Autodesk Inventor part; units mm, degrees
ref_plane "YZ Plane" through (0, 0, 0) normal (1, 0, 0) x (0, 1, 0)
ref_plane "XZ Plane" through (0, 0, 0) normal (0, 1, 0) x (-1, 0, 0)
ref_plane "XY Plane" through (0, 0, 0) normal (0, 0, 1) x (1, 0, 0)
sketch "Sketch2" plane through (0, 0, 0) normal (0, 1, 0) x (-1, 0, 0)
  line L0 (0, 0) -> (-800, 0)
  line L1 (-800, 0) -> (-800, -600)
  line L2 (-800, -600) -> (0, -600)
  line L3 (0, -600) -> (0, 0)
  dimension "d4" = 800
  dimension "d5" = 600
extrude "Extrusion2" add sketch "Sketch2" along normal blind 18
sketch "Sketch3" plane through (0, 0, 0) normal (0, -1, 0) x (1, 0, 0)
  line L0 (0, -600) -> (0, 0)
  line L1 (800, 0) -> (800, -600)
  line L2 (0, 0) -> (800, 0)
  line L3 (800, 0) -> (800, -50)
  line L4 (800, -50) -> (0, -50)
  line L5 (0, -50) -> (0, 0)
  dimension "d8" = 50
extrude "Extrusion3" add sketch "Sketch3" along normal blind 18
sketch "Sketch4" plane through (0, 0, 0) normal (0, -1, 0) x (1, 0, 0)
  line L0 (0, -600) -> (0, 0)
  line L1 (800, 0) -> (800, -600)
  line L2 (0, -600) -> (800, -600)
  line L3 (800, -600) -> (800, -560)
  line L4 (800, -560) -> (0, -560)
  line L5 (0, -560) -> (0, -600)
  dimension "d11" = 40
extrude "Extrusion4" add sketch "Sketch4" along normal blind 18
equation "\"d5\" = Profundidad"
properties part number "tablero_chico" material "Wood (Birch)"
Here's how the part is built. I have some questions about the finished solid (model axes, mm). A direction names the side the tool comes from. Coordinates: 2 decimals unless noted, no trailing zeros. Loops run counter-clockwise (first coordinate to the right, second up) from the corner with the lowest first, then second, coordinate; pieces in that order, holes last. Notation, with made-up numbers: (8.5, 8) -> (42.5, 8) arc R34 cw to (42.5, 38) -> close; hole circle Ø6 at (55, -31.5). An arc over 180 degrees is marked (long way). Use one line per item in the form item = value. Start each with the question number.
(1) If we section it at B-B (x = 71): Please give me the cut outline in (y, z).
(2) We'd pull the mould along Z, two halves only. Please class faces 1 (the face through (406, -9, -560)), 2 (the face through (394, -18, -25)), 3 (the face through (394, 0, -600)), 4 (the face through (406, 0, -301)): pulls with the +Z half, pulls with the -Z half, needs draft (parallel to the pull), parting line crosses it, or undercut.
(3) Please list where these lines run through material, in increasing order: line 1 along Z through (x, y) = (398, -14.5); line 2 along Y through (x, z) = (88.5, -315).
(4) Will these pins go through, and if not, where does the flat tip stop? pin 1 (10 mm diameter, centred on x = 355, y = -0.5, fed in from +Z); pin 2 (8 mm diameter, centred on x = 222, z = -198, fed in from -Y).
(5) If we section it at A-A (y = -5.5): Please give me the cut outline in (x, z), then the cut area to 3 significant figures.
(6) If we section it at C-C (z = -484): Please give me the cut outline in (x, y).
(7) On a 3-axis mill with a long thin cutter (end or side, diameter ignored), from which of +Z, -Z, +X, -X, +Y, -Y can I reach the whole of each face in a straight line? I mean faces 5 (the face through (406, -9, -50)), 6 (the face through (394, -18, -580)). Say none if no direction works.
Verdict:
q1.outline = (-18, -600) -> (18, -600) -> (18, 0) -> (-18, 0) -> (-18, -50) -> (0, -50) -> (0, -560) -> (-18, -560) -> close
q2.face_1 = undercut
q2.face_2 = needs draft
q2.face_3 = pulls with the -Z half
q2.face_4 = undercut
q3.line_1 = -600 to -560, -50 to 0
q3.line_2 = 0 to 18
q4.pin_1 = 0
q4.pin_2 = 0
q5.outline = (0, -600) -> (800, -600) -> (800, -560) -> (0, -560) -> close; (0, -50) -> (800, -50) -> (800, 0) -> (0, 0) -> close
q5.area = 72,000 mm²
q6.outline = (0, 0) -> (800, 0) -> (800, 18) -> (0, 18) -> close
q7.face_5 = +X, -X, -Y
q7.face_6 = +Z, -Z, +X, -X, -Y
